The listing builds one solid part. Answer for the finished solid, in the listing's coordinates (mm). A direction names the side the tool comes from. Round coordinates to 2 decimals unless told otherwise and drop trailing zeros. Write each loop counter-clockwise with the first axis right and the second up, starting at its lowest first coordinate (ties: lowest second). Pieces come first, ordered by that corner, then holes.
from build123d import *

# Parameters (mm, degrees)
SKETCH1_W           = 168
SKETCH1_H           = 22
BOSS_EXTRUDE1_DEPTH = 17.8
SKETCH8_R           = 2
CUT_EXTRUDE4_DEPTH  = 22
CUT_EXTRUDE2_REACH  = 88.567
SKETCH5_W           = 117
SKETCH5_H           = 6
CUT_EXTRUDE3_DEPTH  = 15.8
BOSS_EXTRUDE2_REACH = 90.164
SKETCH9_W           = 47
SKETCH9_H           = 2
FILLET1_R           = 7


with BuildPart() as part:
    # Sketch1 → Boss-Extrude1 (new body)
    with BuildSketch(Plane(origin=(0, 0, 0), x_dir=(1, 0, 0), z_dir=(0, 1, 0))):
        Rectangle(SKETCH1_W, SKETCH1_H)
    extrude(amount=-BOSS_EXTRUDE1_DEPTH)

    # Sketch8 → Cut-Extrude4 (cut)
    with BuildSketch(Plane.XY.offset(11)):
        with Locations((79.55, -13.35)):
            Circle(SKETCH8_R)
    extrude(amount=-CUT_EXTRUDE4_DEPTH, mode=Mode.SUBTRACT)

    # Cut-Extrude2: up to this face of the body (flat: up to its plane)
    cut_extrude2_end = Plane(part.part.faces().sort_by_distance((0, -17.8, 0))[0])
    # Sketch5 → Cut-Extrude2 (cut, up to the picked face)
    with BuildSketch(Plane(origin=(0, 0, 0), x_dir=(1, 0, 0), z_dir=(0, 1, 0)), mode=Mode.PRIVATE) as cut_extrude2_sk1:
        with Locations((25.5, -8)):
            Rectangle(SKETCH5_W, SKETCH5_H)
    cut_extrude2_tool1 = split(extrude(cut_extrude2_sk1.sketch, amount=-CUT_EXTRUDE2_REACH, mode=Mode.PRIVATE), bisect_by=cut_extrude2_end, keep=Keep.BOTH, mode=Mode.PRIVATE)
    add(cut_extrude2_tool1.solids().sort_by(Axis((25.5, 0, 8), (0, -1, 0)))[0], mode=Mode.SUBTRACT)

    # Sketch6 → Cut-Extrude3 (cut)
    with BuildSketch(Plane.XZ.offset(17.8)):
        Polygon((-82, 9), (-82, -9), (82, -9), (82, 3), (-35, 3), (-35, 9), align=None)
    extrude(amount=-CUT_EXTRUDE3_DEPTH, mode=Mode.SUBTRACT)

    # Boss-Extrude2: up to this face of the body (flat: up to its plane)
    boss_extrude2_end = Plane(part.part.faces().sort_by_distance((-0.387668404, -9.883187228, -9))[0])
    # Sketch9 → Boss-Extrude2 (add, up to the picked face)
    with BuildSketch(Plane(origin=(0, 0, 9), x_dir=(-1, 0, 0), z_dir=(0, 0, -1)), mode=Mode.PRIVATE) as boss_extrude2_sk1:
        with Locations((58.5, -13.3)):
            Rectangle(SKETCH9_W, SKETCH9_H)
    boss_extrude2_tool1 = split(extrude(boss_extrude2_sk1.sketch, amount=BOSS_EXTRUDE2_REACH, mode=Mode.PRIVATE), bisect_by=boss_extrude2_end, keep=Keep.BOTH, mode=Mode.PRIVATE)
    add(boss_extrude2_tool1.solids().sort_by(Axis((-58.5, -13.3, 9), (0, 0, -1)))[0])

    # Fillet1
    # the kernel refuses this fillet: 7 mm, written as the material it takes off along each edge
    with BuildSketch(Plane(origin=(84, -17.8, 22.5), x_dir=(-1, 0, 0), z_dir=(0, 0, -1))) as fillet1_piece_1:
        with BuildLine():
            CenterArc((FILLET1_R, FILLET1_R), FILLET1_R, 180, 90)
            Line((0, FILLET1_R), (0, 0))
            Line((0, 0), (FILLET1_R, 0))
        make_face()
    extrude(amount=51, mode=Mode.SUBTRACT)


solid = part.part
1. A tool of negligible diameter and unlimited length cuts with its end or side. For faces 5 (the face through (-82, -7, 0)), 6 (the face through (78.076, -11.998, 4.014)), 7 (the face through (-58, -14.3, 0)), 8 (the face through (25, -9, 5)), 9 (the face through (-59, -9, 11)), from which of +Z, -Z, +X, -X, +Y, -Y can it reach the whole face along a straight path? Write none if from no direction.
Geometry says:
face 5: none
face 6: +Z, -Z
face 7: -Y
face 8: +Z, +X, +Y, -Y
face 9: +Z, +X, -X, +Y, -Y
2. Given pin 1 (9 mm diameter, centred on x = -51, z = 2, fed in from -Y); pin 2 (3 mm diameter, centred on x = -29.5, y = -12, fed in from +Z); pin 3 (3.5 mm diameter, centred on x = 79.55, y = -13.35, fed in from -Z); pin 4 (1.6 mm diameter, centred on y = -13, z = -5.5, fed in from +X), each flat-ended and moving along its own axis, determine where each tip first touches the part or whether it passes through.
Geometry says:
pin 1: stops at y = -14.3
pin 2: stops at z = 5
pin 3: passes through
pin 4: stops at x = 83.86
3. Section A-A on x = -44 is taken. Determine the outline of the cut face in (y, z), plus the area to 3 significant figures.
Geometry says:
outline: (-17.8, -11) - (0, -11) - (0, 11) - (-17.8, 11) - (-17.8, 9) - (-14.3, 9) - (-14.3, -9) - (-17.8, -9) - close; hole (-12.3, -9) - (-2, -9) - (-2, 9) - (-12.3, 9) - close
area: 143 mm2
4. Section C-C on z = -3 is taken. Determine the outline of the cut face in (x, y), plus the area to 3 significant figures.
Geometry says:
outline: (-84, -17.8) - (-82, -17.8) - (-82, -14.3) - (-35, -14.3) - (-35, -12.3) - (-82, -12.3) - (-82, -2) - (82, -2) - (82, -15.7) arc R7 ccw to (84, -10.8) - (84, 0) - (-84, 0) - close
area: 486 mm2
5. Section D-D on x = 74 is taken. Determine the outline of the cut face in (y, z).
Geometry says:
outline: (-17.8, -11) - (0, -11) - (0, 5) - (-17.8, 5) - (-17.8, 3) - (-2, 3) - (-2, -9) - (-17.8, -9) - close
6. Straight lines are drawn through the part: line 1 along Z through (x, y) = (-55, -4.5); line 2 along Z through (x, y) = (15.5, -11); line 3 along Y through (x, z) = (-59.5, -8.25). For each, find the intervals that lie inside material, in ascending order.
Geometry says:
line 1: z = -11 to -9, 9 to 11
line 2: z = -11 to -9, 3 to 5
line 3: y = -14.3 to -12.3, -2 to 0
7. For a pull along X with two mould halves and no side action, classify faces 1 (the face through (-35, -7, 6)), 2 (the face through (-1, -9, -11)), 3 (the face through (-33, -9, 8)), 4 (the face through (-58, -12.3, 0)) as released by +X, released by -X, zero draft, split by the parting line, or undercut.
Geometry says:
face 1: undercut
face 2: zero draft
face 3: released by +X
face 4: undercut
8. Section B-B on y = -4 is taken. Determine the outline of the cut face in (x, z), plus the area to 3 significant figures.
Geometry says:
outline: (-84, -11) - (84, -11) - (84, 5) - (-33, 5) - (-33, 11) - (-84, 11) - close; hole (-82, -9) - (82, -9) - (82, 3) - (-35, 3) - (-35, 9) - (-82, 9) - close
area: 744 mm2
